The listing builds one solid part. Answer for the finished solid, in the listing's coordinates (mm). A direction names the side the tool comes from. Give positions to 0.01 mm unless a question says otherwise; leave off trailing zeros. Write each loop counter-clockwise with the first axis right and the second up, starting at its lowest first coordinate (ties: lowest second). Pieces come first, ordered by that corner, then holes. Notation, with made-up numbers: (-33, -31) - (26, -31) arc R17 cw to (26, -3) - close; hole circle Ø1 at (-27, -15.75). An arc over 180 degrees is marked (long way). Return JSON: item names as keys, results as strings.
from build123d import *

# Parameters (mm, degrees)
EXTRUDE_1_DEPTH     = 22
SKETCH_2_R          = 2.55
CUT_EXTRUDE_1_DEPTH = 61.497933849
FILLET_1_R          = 8


with BuildPart() as part:
    # Эскиз1 → Бобышка-Вытянуть1 (new body)
    with BuildSketch(Plane(origin=(0, 0, 0), x_dir=(0, 0, -1), z_dir=(1, 0, 0))):
        with BuildLine():
            Line((10.206185567, 0), (10.206185567, -40))
            Line((10.206185567, -40), (13.206185567, -40))
            Line((13.206185567, -40), (13.206185567, 50))
            Line((13.206185567, 50), (10.206185567, 50))
            Line((10.206185567, 50), (10.206185567, 16))
            ThreePointArc((10.206185567, 16), (7.863039817, 10.343145751), (2.206185567, 8))
            Line((2.206185567, 8), (-1.793814433, 8))
            ThreePointArc((-1.793814433, 8), (-7.450668682, 10.343145751), (-9.793814433, 16))
            Line((-9.793814433, 16), (-9.793814433, 50))
            Line((-9.793814433, 50), (-12.793814433, 50))
            Line((-12.793814433, 50), (-12.793814433, -40))
            Line((-12.793814433, -40), (-9.793814433, -40))
            Line((-9.793814433, -40), (-9.793814433, 0))
            Line((-9.793814433, 0), (10.206185567, 0))
        make_face()
    extrude(amount=EXTRUDE_1_DEPTH)

    # Эскиз2 → Вырез-Вытянуть1 (cut, through all)
    with BuildSketch(Plane.XY.offset(12.793814433)):
        with Locations((11, -30)):
            Circle(SKETCH_2_R)
        with Locations((11, -10)):
            Circle(SKETCH_2_R)
        with Locations((11, 39)):
            Circle(SKETCH_2_R)
    extrude(amount=-CUT_EXTRUDE_1_DEPTH, mode=Mode.SUBTRACT)

    # Скругление1
    fillet_1_edges = [part.edges().sort_by_distance(p)[0] for p in [
        (22, -40, -11.706185567),
        (0, -40, 11.293814433),
        (0, 50, 11.293814433),
        (22, 50, -11.706185567),
        (0, 50, -11.706185567),
        (0, -40, -11.706185567),
        (22, 50, 11.293814433),
        (22, -40, 11.293814433),
    ]]
    fillet(fillet_1_edges, radius=FILLET_1_R)


solid = part.part
Item 1: A cutting plane is placed at B-B on y = -30. Determine the outline of the cut face in (x, z), then the cut area to 3 significant figures.
Answer below:
{"outline": "(0, -13.21) - (8.45, -13.21) - (8.45, -10.21) - (0, -10.21) - close; (0, 9.79) - (8.45, 9.79) - (8.45, 12.79) - (0, 12.79) - close; (13.55, -13.21) - (22, -13.21) - (22, -10.21) - (13.55, -10.21) - close; (13.55, 9.79) - (22, 9.79) - (22, 12.79) - (13.55, 12.79) - close", "area": "101 mm²"}
Item 2: For faces 1 (the face through (11, -20, 9.794)), 2 (the face through (10.846, 10.281, 7.388)), 3 (the face through (0, 5, -1)), determine the directions among +Z, -Z, +X, -X, +Y, -Y from which every point of the face is accessible in a straight line to the end or side of a thin tool.
Answer below:
{"face 1": "+X, -X, -Y", "face 2": "+X, -X, +Y", "face 3": "+Z, -Z, -X, +Y, -Y"}
Item 3: A cutting plane is placed at D-D on x = 11. Give the number of separate pieces and of enclosed holes in the cut face, then the cut area to 3 significant figures.
Answer below:
{"separate pieces": "7", "enclosed holes": "0", "area": "636 mm²"}
Item 4: A cutting plane is placed at A-A on y = 23.5. Determine the outline of the cut face in (x, z).
Answer below:
{"outline": "(0, -13.21) - (22, -13.21) - (22, -10.21) - (0, -10.21) - close; (0, 9.79) - (22, 9.79) - (22, 12.79) - (0, 12.79) - close"}
Item 5: Consider L1, parallel to Y at x = 11, z = 11.1; L2, parallel to Z at x = 9.5, y = -26; L3, parallel to Y at x = 2.5, z = -7.25. Determine where each line is inside the solid, lowest interval first.
Answer below:
{"L1": "y = -40 to -32.55, -27.45 to -12.55, -7.45 to 36.45, 41.55 to 50", "L2": "z = -13.21 to -10.21, 9.79 to 12.79", "L3": "y = 0 to 9.79"}
Item 6: The mould has two halves that part along Z. Classify faces 4 (the face through (11, 0, 0)), 5 (the face through (10.67, -27.47, -11.69)), 6 (the face through (11, 6, 12.794)): +Z half, -Z half, draft (parallel to the pull), parting line (faces both ways), or undercut.
Answer below:
{"face 4": "undercut", "face 5": "draft", "face 6": "+Z half"}
Item 7: A cutting plane is placed at C-C on x = 20.25. Determine the outline of the cut face in (y, z).
Answer below:
{"outline": "(-36.99, -13.21) - (46.99, -13.21) - (46.99, -10.21) - (16, -10.21) arc R8 cw to (8, -2.21) - (8, 1.79) arc R8 cw to (16, 9.79) - (46.99, 9.79) - (46.99, 12.79) - (-36.99, 12.79) - (-36.99, 9.79) - (0, 9.79) - (0, -10.21) - (-36.99, -10.21) - close"}
Item 8: Flat-ended cylindrical pins translate along their axes: P1, Ø10, axis at x = 16, z = -2.5, coming from the -Y side; P2, Ø8, axis at x = 2.5, z = -1.5, coming from the +Y side; P3, Ø2, axis at x = 6, z = -1, coming from the +Y side. Find the tip coordinate at first contact, or state that the pin passes through.
Answer below:
{"P1": "stops at y = 0", "P2": "stops at y = 8.71", "P3": "stops at y = 8"}
